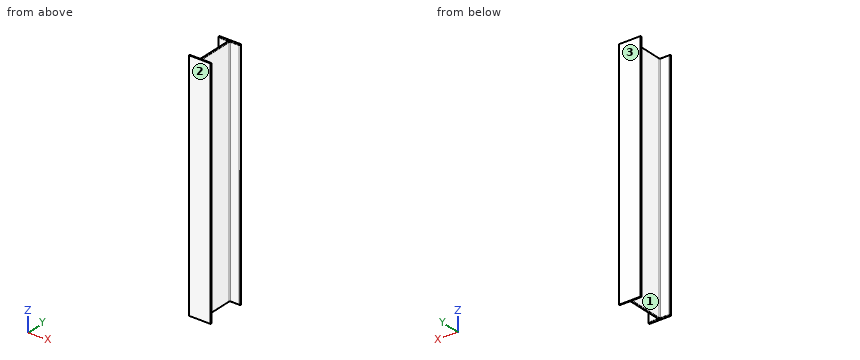
```python
from build123d import *

# Parameters (mm, degrees)
BOSS_EXTRUDE1_DEPTH = 457.2
FILLET1_R           = 2.921


with BuildPart() as part:
    # Sketch1 → Boss-Extrude1 (new, symmetric)
    with BuildSketch(Plane.XY):
        Polygon((42.291, 152.4), (-42.291, 152.4), (-42.291, 146.558), (-2.921, 146.558), (-2.921, 5.842), (-42.291, 5.842), (-42.291, 0), (42.291, 0), (42.291, 5.842), (2.921, 5.842), (2.921, 146.558), (42.291, 146.558), align=None)
    extrude(amount=BOSS_EXTRUDE1_DEPTH, both=True)

    # Fillet1
    fillet1_edges = [part.edges().sort_by_distance(p)[0] for p in [
        (22.606, 146.558, -457.2),
        (2.921, 76.2, -457.2),
        (22.606, 5.842, -457.2),
        (-22.606, 146.558, 457.2),
        (-22.606, 5.842, -457.2),
        (-2.921, 76.2, -457.2),
        (-22.606, 146.558, -457.2),
        (-2.921, 76.2, 457.2),
        (-22.606, 5.842, 457.2),
        (42.291, 146.558, 0),
        (2.921, 146.558, 0),
        (2.921, 5.842, 0),
        (42.291, 5.842, 0),
        (-42.291, 5.842, 0),
        (-2.921, 5.842, 0),
        (-2.921, 146.558, 0),
        (-42.291, 146.558, 0),
        (22.606, 5.842, 457.2),
        (2.921, 76.2, 457.2),
        (22.606, 146.558, 457.2),
    ]]
    fillet(fillet1_edges, radius=FILLET1_R - 0.0001)  # a hair under: the kernel refuses the full size


solid = part.part
```
Check sheet for the modelled part. Datum: model origin and axes. Units: mm. Face numbers are marked on the shaded views. Coordinates: 2 decimals unless noted, no trailing zeros. Loops run counter-clockwise (first coordinate to the right, second up) from the corner with the lowest first, then second, coordinate; pieces in that order, holes last.
1) Release check for a two-part mould opening along Y. For the marked faces 1, 2 and 3 record: released by +Y, released by -Y, zero draft, split by the parting line, or undercut.
2) Sectioned sample at A-A (x = 19.5). Record the boundary of the cut face in (y, z).
3) Sectioned sample at B-B (z = 287). Record the boundary of the cut face in (x, y), and give its area (3 significant figures).
4) Gauge pin test, flat end, axial feed: pin 1 (1 mm diameter, centred on y = 54, z = 293.5, fed in from +X). Record the tip position at first contact, or that the pin passes through.
5) Material ranges on probe 1 along Y at (x, z) = (-16.5, -83); probe 2 along X at (y, z) = (103, 214); probe 3 along Y at (x, z) = (-5.5, -3), recorded low to high.
Check sheet entries:
1. face 1: undercut
1. face 2: released by -Y
1. face 3: released by +Y
2. outline: (0, -457.2) - (2.92, -457.2) arc R2.92 ccw to (5.84, -454.28) - (5.84, 454.28) arc R2.92 ccw to (2.92, 457.2) - (0, 457.2) - close; (146.56, -454.28) arc R2.92 ccw to (149.48, -457.2) - (152.4, -457.2) - (152.4, 457.2) - (149.48, 457.2) arc R2.92 ccw to (146.56, 454.28) - close
3. outline: (-42.29, 0) - (42.29, 0) - (42.29, 2.92) arc R2.92 ccw to (39.37, 5.84) - (5.84, 5.84) arc R2.92 cw to (2.92, 8.76) - (2.92, 143.64) arc R2.92 cw to (5.84, 146.56) - (39.37, 146.56) arc R2.92 ccw to (42.29, 149.48) - (42.29, 152.4) - (-42.29, 152.4) - (-42.29, 149.48) arc R2.92 ccw to (-39.37, 146.56) - (-5.84, 146.56) arc R2.92 cw to (-2.92, 143.64) - (-2.92, 8.76) arc R2.92 cw to (-5.84, 5.84) - (-39.37, 5.84) arc R2.92 ccw to (-42.29, 2.92) - close
3. area: 1,810 mm2
4. pin 1: stops at x = 2.92
5. probe 1: y = 0 to 5.84, 146.56 to 152.4
5. probe 2: x = -2.92 to 2.92
5. probe 3: y = 0 to 5.86, 146.54 to 152.4
